Read the model definition and answer for the solid it produces. Units are mm, in the model's axes. Face numbers are marked on the shaded views. A direction names the side the tool comes from. Coordinates: 2 decimals unless noted, no trailing zeros. Loops run counter-clockwise (first coordinate to the right, second up) from the corner with the lowest first, then second, coordinate; pieces in that order, holes last. Notation, with made-up numbers: (45, 47) -> (82, 47) arc R24 ccw to (82, 71) -> close; hole circle Ø7 at (86, -2.5). An arc over 180 degrees is marked (long way). Answer as CSV lines item,"result".
```python
from build123d import *

# Parameters (mm, degrees)
F0_R     = 1.5
F0_R_2   = 13.6669430684
F1_DEPTH = 3
F2_DEPTH = 42


# Not quite as in the source:
# - a feature names something its author has since deleted; it is built from what else it names


with BuildPart() as f1:
    # F0 (on Top) → F1 (new body)
    with BuildSketch(Plane.XY):
        Polygon((21, 21), (-21, 21), (-21, -21), (-3.25, -21), (0, -21), (3.25, -21), (21, -21), align=None)
        with Locations((-15.5, -15.5)):
            Circle(F0_R, mode=Mode.SUBTRACT)
        with Locations((-15.5, 15.5)):
            Circle(F0_R, mode=Mode.SUBTRACT)
        Circle(F0_R_2, mode=Mode.SUBTRACT)
        with Locations((15.5, -15.5)):
            Circle(F0_R, mode=Mode.SUBTRACT)
        with Locations((15.5, 15.5)):
            Circle(F0_R, mode=Mode.SUBTRACT)
    extrude(amount=F1_DEPTH)

    # F0 (on Top) → F2 (join)
    with BuildSketch(Plane.XY):
        Polygon((12.5, -44.75), (15.25, -44.75), (15.25, -38.25), (12.5, -38.25), (12.5, -31.125), (7.75, -36), (7.75, -41.5), (7.75, -47), (12.5, -51.875), align=None)
        Polygon((-3.25, -21), (-21, -21), (-21, -26.5), (-21, -56.5), (-15.25, -56.5), (-15.25, -44.75), (-15.25, -38.25), (-15.25, -26.5), (-3.75, -26.5), (0, -26.5), (3.75, -26.5), (15.25, -26.5), (15.25, -38.25), (15.25, -44.75), (15.25, -56.5), (21, -56.5), (21, -26.5), (21, -21), (3.25, -21), (0, -21), align=None)
        Polygon((0, -26.5), (-3.75, -26.5), (-3.75, -29), (-10.875, -29), (-5.5, -33.75), (0, -33.75), (5.5, -33.75), (10.875, -29), (3.75, -29), (3.75, -26.5), align=None)
        Polygon((-15.25, -38.25), (-15.25, -44.75), (-12.5, -44.75), (-12.5, -51.875), (-7.75, -47), (-7.75, -41.5), (-7.75, -36), (-12.5, -31.125), (-12.5, -38.25), align=None)
    extrude(amount=F2_DEPTH)


solid = f1.part
```
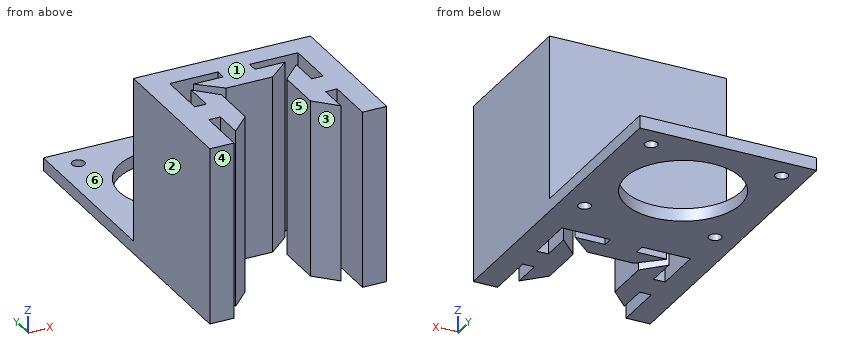
Q1. A cutting plane is placed at A-A, the plane y = 0. Write down the section's boundary in (x, z), and give its area (3 significant figures).
Results:
outline,"(-21, 0) -> (-13.67, 0) -> (-13.67, 3) -> (-21, 3) -> close; (13.67, 0) -> (21, 0) -> (21, 3) -> (13.67, 3) -> close"
area,"44.0 mm²"
Q2. A cutting plane is placed at D-D, the plane x = -6.5. Write down the section's boundary in (y, z), and give its area (3 significant figures).
Results:
outline,"(-32.87, 0) -> (-29, 0) -> (-29, 42) -> (-32.87, 42) -> close; (-26.5, 0) -> (-12.02, 0) -> (-12.02, 3) -> (-21, 3) -> (-21, 42) -> (-26.5, 42) -> close; (12.02, 0) -> (21, 0) -> (21, 3) -> (12.02, 3) -> close"
area,"447 mm²"
Q3. For a pull along X with two mould halves and no side action, classify the marked faces 1, 2 and 3 as pulls with the +X half, pulls with the -X half, needs draft (parallel to the pull), parting line crosses it, or undercut.
Results:
face 1,"needs draft"
face 2,"pulls with the -X half"
face 3,"undercut"
Q4. Given pin 1 Ø4 at (x, z) = (-0.5, 22.5) entering from -Y; pin 2 Ø2.5 at (x, y) = (-15.5, -15.5) entering from -Z; pin 3 Ø1.4 at (x, z) = (-14, 23) entering from -Y; pin 4 Ø3 at (x, z) = (14.5, 18) entering from +Y, each flat-ended and moving along its own axis, determine where each tip first touches the part or whether it passes through.
Results:
pin 1,"stops at y = -33.75"
pin 2,"passes through"
pin 3,"stops at y = -44.75"
pin 4,"stops at y = -21"
Q5. For the marked faces 4, 5 and 6, determine the directions among +Z, -Z, +X, -X, +Y, -Y from which every point of the face is accessible in a straight line to the end or side of a thin tool.
Results:
face 4,"+Z, -Z, +X, -X, -Y"
face 5,"+Z, -Z, -Y"
face 6,"+Z, +X, -X, +Y"
Q6. A cutting plane is placed at C-C, the plane y = 15.5. Write down the section's boundary in (x, z), and give its area (3 significant figures).
Results:
outline,"(-21, 0) -> (-17, 0) -> (-17, 3) -> (-21, 3) -> close; (-14, 0) -> (14, 0) -> (14, 3) -> (-14, 3) -> close; (17, 0) -> (21, 0) -> (21, 3) -> (17, 3) -> close"
area,"108 mm²"
Q7. Find the intervals of material crossed by probe 1 along Y at (x, z) = (15.5, 1.3); probe 2 along Y at (x, z) = (0, 0.85); probe 3 along X at (y, z) = (-48, 16.5), in increasing order. Write a range as [from, to].
Results:
probe 1,"y = [-56.5, -17], [-14, 14], [17, 21]"
probe 2,"y = [-33.75, -13.67], [13.67, 21]"
probe 3,"x = [-21, -15.25], [-12.5, -8.72], [8.72, 12.5], [15.25, 21]"
Q8. A cutting plane is placed at B-B, the plane y = -37. Write down the section's boundary in (x, z).
Results:
outline,"(-21, 0) -> (-15.25, 0) -> (-15.25, 42) -> (-21, 42) -> close; (-12.5, 0) -> (-7.75, 0) -> (-7.75, 42) -> (-12.5, 42) -> close; (7.75, 0) -> (12.5, 0) -> (12.5, 42) -> (7.75, 42) -> close; (15.25, 0) -> (21, 0) -> (21, 42) -> (15.25, 42) -> close"
